from build123d import *

# Parameters (mm, degrees)
SKETCH2_OUTSIDE_W  = 48.751
SKETCH2_OUTSIDE_H  = 48.752
CUT_EXTRUDE1_DEPTH = 79.163904494


with BuildPart() as part:
    # Sketch1 → Revolve1 (revolve)
    with BuildSketch(Plane.XY):
        with BuildLine():
            Line((13.945442694, -14.186787019), (13.945442694, -1.101180597))
            Line((13.945442694, -1.101180597), (13.945442694, 49.313212981))
            Line((13.945442694, 49.313212981), (20.295442694, 49.313212981))
            Line((20.295442694, 49.313212981), (20.295442694, -18.555587019))
            Line((20.295442694, -18.555587019), (7.413252884, -18.555587019))
            ThreePointArc((7.413252884, -18.555587019), (6.158112274, -17.849568811), (4.972892694, -17.031587019))
            Line((4.972892694, -17.031587019), (4.972892694, -14.186787019))
            Line((4.972892694, -14.186787019), (13.945442694, -14.186787019))
        make_face()
    revolve(axis=Axis((20.295442694, 49.313212981, 0), (0, -1, 0)))

    # Sketch2 outside → Cut-Extrude1 (cut, through all)
    with BuildSketch(Plane.XZ.offset(18.555587019)):
        with Locations((20.2955, 0)):
            Rectangle(SKETCH2_OUTSIDE_W, SKETCH2_OUTSIDE_H)
        Polygon((20.295442694, 15.322011053), (7.026191885, 7.661005527), (7.026191885, -7.661005527), (20.295442694, -15.322011053), (33.564693504, -7.661005527), (33.564693504, 7.661005527), align=None, mode=Mode.SUBTRACT)
    extrude(amount=-CUT_EXTRUDE1_DEPTH, mode=Mode.SUBTRACT)


solid = part.part
Verification items for the finished model (mm, model axes). A direction names the side the tool comes from. Coordinates: 2 decimals unless noted, no trailing zeros. Write each loop counter-clockwise with the first axis right and the second up, starting at its lowest first coordinate (ties: lowest second). Pieces come first, ordered by that corner, then holes. Notation, with made-up numbers: (18, 46.5) -> (32, 46.5) arc R36 cw to (32, 85.5) -> close; hole circle Ø2 at (88.5, -15). An arc over 180 degrees is marked (long way). One line per item, written item: value. Start each with the question number.
Q1. Go/stop test with flat-tipped pins: P1, Ø4, axis at x = 10.5, y = 12.5, coming from the -Z side; P2, Ø6, axis at x = 27.5, y = -7.5, coming from the -Z side; P3, Ø8, axis at x = 14.5, y = 1.5, coming from the -Z side; P4, Ø10, axis at y = 27, z = -0.5, coming from the -X side. Record where each tip stops, or that it passes through.
Q2. Thickness scan on L1, parallel to Y at x = 25.5, z = 10; L2, parallel to X at y = 37.5, z = 5.5; L3, parallel to Z at x = 24.25, y = 43.5. Record the ranges inside material, lowest first. Write a range as from..to.
Q3. Access from +Z, -Z, +X, -X, +Y, -Y to the whole of each face (thin tool, end or side, straight path). Record for faces 1 (the flat face through (20, 49.313, 0)), 2 (the flat face through (20, -14.187, 7)).
Q4. Cross-section at A-A on y = 12. Enter the section's corners in (x, z), and give its area (3 significant figures).
Checked values:
1. P1: passes through
1. P2: stops at z = -4.76
1. P3: stops at z = -6.09
1. P4: stops at x = 13.95
2. L1: y = -18.56..-14.19
2. L2: x = 17.12..23.47
2. L3: z = -4.97..4.97
3. face 1: +Z, -Z, +X, -X, +Y
3. face 2: +Y
4. outline: circle Ø12.7 at (20.3, 0)
4. area: 127 mm²
